```python
from build123d import *

# Parameters (mm, degrees)
SKETCH1_R           = 5
SKETCH1_W           = 22
SKETCH1_H           = 11
BOSS_EXTRUDE1_DEPTH = 8


with BuildPart() as part:
    # Sketch1 → Boss-Extrude1 (new body)
    with BuildSketch(Plane.XY):
        with BuildLine():
            Line((75, -7.5), (-75, -7.5))
            ThreePointArc((-75, -7.5), (-82.5, 0), (-75, 7.5))
            Line((-75, 7.5), (75, 7.5))
            ThreePointArc((75, 7.5), (82.5, 0), (75, -7.5))
        make_face()
        with Locations((75, 0)):
            Circle(SKETCH1_R, mode=Mode.SUBTRACT)
        with Locations(Location((-75, 0, 0), (0, 0, 180))):
            Circle(SKETCH1_R, mode=Mode.SUBTRACT)
        with Locations((-5, 0)):
            Rectangle(SKETCH1_W, SKETCH1_H, mode=Mode.SUBTRACT)
    extrude(amount=BOSS_EXTRUDE1_DEPTH)


solid = part.part
```
Verification items for the finished model (mm, model axes). A direction names the side the tool comes from. Round coordinates to 2 decimals unless told otherwise and drop trailing zeros. Order: outer loops, then holes, each group sorted by start corner. A loop starts at its lowest first (then second) coordinate and runs counter-clockwise, first axis right, second up. Notation, with made-up numbers: (32.25, 4.25) -> (86.25, 4.25) arc R27 ccw to (86.25, 37.25) -> close; hole circle Ø2 at (79.5, -36.5). An arc over 180 degrees is marked (long way). Put each result on its own line as item: value. Start each with the question number.
(1) Section check C-C (z = 5.5). Enter the section's corners in (x, y).
(2) Tool access check on faces 1 (the face through (1, -7.5, 4)), 2 (the face through (6, 0, 4)). Record the directions out of +Z, -Z, +X, -X, +Y, -Y that give a thin tool (end or side, any length) a straight path to the whole face; none if there is none.
(3) Draft check along Y on faces 3 (the face through (1, 7, 8)), 4 (the face through (-79.619, 1.915, 3.944)), 5 (the face through (82.5, 0.16, 3.94)). Enter one of: +Y half, -Y half, draft (parallel to the pull), parting line (faces both ways), or undercut.
(4) Material ranges on line 1 along X through (y, z) = (-1.25, 3); line 2 along X through (y, z) = (-2.75, 2); line 3 along Y through (x, z) = (-75, 2), recorded low to high.
(5) Section check A-A (x = -13). Enter the section's corners in (y, z).
(6) Section check B-B (y = 0). Enter the section's corners in (x, z).
(7) Depth check by flat-ended pin: pin 1 Ø1 at (y, z) = (-2, 7) entering from +X; pin 2 Ø2 at (y, z) = (2.5, 3) entering from -X. Enter the tip coordinate at first touch or a pass-through.
Completed:
1. outline: (-75, -7.5) -> (75, -7.5) arc R7.5 ccw to (75, 7.5) -> (-75, 7.5) arc R7.5 ccw to start; hole circle Ø10 at (-75, 0); hole (-16, -5.5) -> (6, -5.5) -> (6, 5.5) -> (-16, 5.5) -> close; hole circle Ø10 at (75, 0)
2. face 1: +Z, -Z, +X, -X, -Y
2. face 2: +Z, -Z
3. face 3: draft
3. face 4: undercut
3. face 5: parting line
4. line 1: x = -82.4 to -79.84, -70.16 to -16, 6 to 70.16, 79.84 to 82.4
4. line 2: x = -81.98 to -79.18, -70.82 to -16, 6 to 70.82, 79.18 to 81.98
4. line 3: y = -7.5 to -5, 5 to 7.5
5. outline: (-7.5, 0) -> (-5.5, 0) -> (-5.5, 8) -> (-7.5, 8) -> close; (5.5, 0) -> (7.5, 0) -> (7.5, 8) -> (5.5, 8) -> close
6. outline: (-82.5, 0) -> (-80, 0) -> (-80, 8) -> (-82.5, 8) -> close; (-70, 0) -> (-16, 0) -> (-16, 8) -> (-70, 8) -> close; (6, 0) -> (70, 0) -> (70, 8) -> (6, 8) -> close; (80, 0) -> (82.5, 0) -> (82.5, 8) -> (80, 8) -> close
7. pin 1: stops at x = 82.35
7. pin 2: stops at x = -82.35
